from build123d import *

# Parameters (mm, degrees)
SKETCH1_W           = 150
SKETCH1_H           = 100
SKETCH1_H_2         = 400
SKETCH1_W_2         = 15
SKETCH1_H_3         = 25
SKETCH1_W_3         = 30
BOSS_EXTRUDE1_DEPTH = 4
BOSS_EXTRUDE2_START = 4
SKETCH1_4_W         = 15
SKETCH1_4_H         = 25
SKETCH1_4_W_2       = 30
BOSS_EXTRUDE2_DEPTH = 10
BOSS_EXTRUDE3_START = 14
SKETCH1_5_W         = 30
SKETCH1_5_H         = 50
BOSS_EXTRUDE3_DEPTH = 60
BOSS_EXTRUDE4_START = 4
SKETCH15_W          = 40
SKETCH15_H          = 15
BOSS_EXTRUDE4_DEPTH = 70
SKETCH16_R          = 5.2
CUT_EXTRUDE1_DEPTH  = 588.772064665
CUT_EXTRUDE2_START  = 300
SKETCH17_W          = 20
SKETCH17_H          = 20
CUT_EXTRUDE2_DEPTH  = 26
CUT_EXTRUDE3_START  = 270
CUT_EXTRUDE3_DEPTH  = 318.772064665


with BuildPart() as part:
    # Sketch1 → Boss-Extrude1 (new body)
    with BuildSketch(Plane(origin=(0, 0, 0), x_dir=(1, 0, 0), z_dir=(0, 1, 0))):
        with Locations((75, 50)):
            Rectangle(SKETCH1_W, SKETCH1_H)
        with Locations((75, 300)):
            Rectangle(SKETCH1_W, SKETCH1_H_2)
        Polygon((300, 500), (150, 500), (150, 100), (255, 100), (255, 125), (270, 125), (300, 125), align=None)
        with Locations((262.5, 112.5)):
            Rectangle(SKETCH1_W_2, SKETCH1_H_3)
        with Locations((285, 112.5)):
            Rectangle(SKETCH1_W_3, SKETCH1_H_3)
        Polygon((255, 100), (150, 100), (150, 0), (300, 0), (300, 75), (270, 75), (255, 75), align=None)
        with Locations((262.5, 87.5)):
            Rectangle(SKETCH1_W_2, SKETCH1_H_3)
        with Locations((285, 87.5)):
            Rectangle(SKETCH1_W_3, SKETCH1_H_3)
    extrude(amount=BOSS_EXTRUDE1_DEPTH)

    # Sketch1<4> → Boss-Extrude2 (add)
    with BuildSketch(Plane(origin=(0, 0, 0), x_dir=(1, 0, 0), z_dir=(0, 1, 0)).offset(BOSS_EXTRUDE2_START)):
        with Locations((262.5, 112.5)):
            Rectangle(SKETCH1_4_W, SKETCH1_4_H)
        with Locations((262.5, 87.5)):
            Rectangle(SKETCH1_4_W, SKETCH1_4_H)
        with Locations((285, 87.5)):
            Rectangle(SKETCH1_4_W_2, SKETCH1_4_H)
        with Locations((285, 112.5)):
            Rectangle(SKETCH1_4_W_2, SKETCH1_4_H)
    extrude(amount=BOSS_EXTRUDE2_DEPTH)

    # Sketch1<5> → Boss-Extrude3 (add)
    with BuildSketch(Plane(origin=(0, 0, 0), x_dir=(1, 0, 0), z_dir=(0, 1, 0)).offset(BOSS_EXTRUDE3_START)):
        with Locations((285, 100)):
            Rectangle(SKETCH1_5_W, SKETCH1_5_H)
    extrude(amount=BOSS_EXTRUDE3_DEPTH)

    # Sketch15 → Boss-Extrude4 (add)
    with BuildSketch(Plane(origin=(0, 0, 0), x_dir=(1, 0, 0), z_dir=(0, 1, 0)).offset(BOSS_EXTRUDE4_START)):
        with Locations((225, 122.5)):
            Rectangle(SKETCH15_W, SKETCH15_H)
        with Locations((225, 77.5)):
            Rectangle(SKETCH15_W, SKETCH15_H)
        with Locations((45, 135.366666062)):
            Rectangle(SKETCH15_W, SKETCH15_H)
    extrude(amount=BOSS_EXTRUDE4_DEPTH)

    # Sketch16 → Cut-Extrude1 (cut, through all)
    with BuildSketch(Plane.XY):
        with Locations((225, 54)):
            Circle(SKETCH16_R)
        with Locations((45, 54)):
            Circle(SKETCH16_R)
    extrude(amount=-CUT_EXTRUDE1_DEPTH, mode=Mode.SUBTRACT)

    # Sketch17 → Cut-Extrude2 (cut)
    with BuildSketch(Plane(origin=(0, 0, 0), x_dir=(0, 0, -1), z_dir=(1, 0, 0)).offset(CUT_EXTRUDE2_START)):
        with Locations((100, 54)):
            Rectangle(SKETCH17_W, SKETCH17_H)
    extrude(amount=-CUT_EXTRUDE2_DEPTH, mode=Mode.SUBTRACT)

    # Sketch17<3> → Cut-Extrude3 (cut, through all)
    with BuildSketch(Plane(origin=(0, 0, 0), x_dir=(0, 0, -1), z_dir=(1, 0, 0)).offset(CUT_EXTRUDE3_START)):
        with BuildLine():
            ThreePointArc((103.25, 54), (102.298097039, 56.298097039), (100, 57.25))
            Line((100, 57.25), (100, 50.75))
            ThreePointArc((100, 50.75), (102.298097039, 51.701902961), (103.25, 54))
        make_face()
        with BuildLine():
            Line((100, 50.75), (100, 57.25))
            ThreePointArc((100, 57.25), (96.75, 54), (100, 50.75))
        make_face()
    extrude(amount=CUT_EXTRUDE3_DEPTH, mode=Mode.SUBTRACT)


solid = part.part
Read the model definition and answer for the solid it produces. Units are mm, in the model's axes. A direction names the side the tool comes from. Give positions to 0.01 mm unless a question says otherwise; leave off trailing zeros. Write each loop counter-clockwise with the first axis right and the second up, starting at its lowest first coordinate (ties: lowest second). Pieces come first, ordered by that corner, then holes. Notation, with made-up numbers: (-9, 57) - (11, 57) arc R34 ccw to (11, 90) - close; hole circle Ø8 at (25.5, -26.5). An arc over 180 degrees is marked (long way). Use CSV: the item, a comma, the result in double quotes. Start each with the question number.
Item 1: The part is cut by section B-B, the plane y = 27.5. Give the vertices of the cut face in (x, z), and give its area (3 significant figures).
Item 2: Flat-ended cylindrical pins translate along their axes: P1, Ø5, axis at x = 60, y = 7.5, coming from the -Z side; P2, Ø8, axis at y = 9, z = -112, coming from the -X side; P3, Ø22, axis at x = 292, y = 56, coming from the -Z side. Find the tip coordinate at first contact, or state that the pin passes through.
Item 3: The mould has two halves that part along Z. Classify faces 6 (the flat face through (287, 44, -100)), 7 (the flat face through (225, 74, -78)), 8 (the flat face through (45, 39, -127.867)), 9 (the flat face through (225, 39, -115)): pulls with the +Z half, pulls with the -Z half, needs draft (parallel to the pull), parting line crosses it, or undercut.
Item 4: The part is cut by section D-D, the plane z = -403.5. Give the vertices of the cut face in (x, y), and give its area (3 significant figures).
Item 5: The part is cut by section C-C, the plane x = 225. Give the vertices of the cut face in (y, z).
Item 6: The part is cut by section A-A, the plane x = 45. Give the vertices of the cut face in (y, z), and give its area (3 significant figures).
Item 7: Consider line 1 (Y direction, x = 225, z = -74.5); line 2 (X direction, y = 51, z = -120.5); line 3 (Y direction, x = 19.5, z = -444). Determine where each line is inside the solid, lowest interval first.
Item 8: For faces 1 (the flat face through (282, 39, -75)), 2 (the flat face through (45, 39, -142.867)), 3 (the flat face through (255, 9, -100)), 4 (the flat face through (25, 39, -135)), 5 (the flat face through (287, 54, -110)), determine the directions among +Z, -Z, +X, -X, +Y, -Y from which every point of the face is accessible in a straight line to the end or side of a thin tool.
Taken from the geometry:
1,outline,"(25, -142.87) - (65, -142.87) - (65, -127.87) - (25, -127.87) - close; (205, -130) - (245, -130) - (245, -115) - (205, -115) - close; (205, -85) - (245, -85) - (245, -70) - (205, -70) - close; (270, -125) - (300, -125) - (300, -75) - (270, -75) - close"
1,area,"3,300 mm2"
2,P1,"z = -142.87"
2,P2,"x = 205"
2,P3,"z = -125"
3,face 6,"undercut"
3,face 7,"needs draft"
3,face 8,"pulls with the +Z half"
3,face 9,"undercut"
4,outline,"(0, 0) - (300, 0) - (300, 4) - (0, 4) - close"
4,area,"1,200 mm2"
5,outline,"(0, -500) - (4, -500) - (4, -130) - (48.8, -130) - (48.8, -115) - (4, -115) - (4, -85) - (48.8, -85) - (48.8, -70) - (4, -70) - (4, 0) - (0, 0) - close; (59.2, -130) - (74, -130) - (74, -115) - (59.2, -115) - close; (59.2, -85) - (74, -85) - (74, -70) - (59.2, -70) - close"
6,outline,"(0, -500) - (4, -500) - (4, -142.87) - (48.8, -142.87) - (48.8, -127.87) - (4, -127.87) - (4, 0) - (0, 0) - close; (59.2, -142.87) - (74, -142.87) - (74, -127.87) - (59.2, -127.87) - close"
6,area,"2,890 mm2"
7,line 1,"0 to 48.8, 59.2 to 74"
7,line 2,"205 to 220.75, 229.25 to 245, 270 to 300"
7,line 3,"0 to 4"
8,face 1,"+Z, +X, +Y"
8,face 2,"-Z, +X, -X, +Y"
8,face 3,"+Z, -Z, +Y"
8,face 4,"+Z, -Z, -X, +Y"
8,face 5,"+X"
